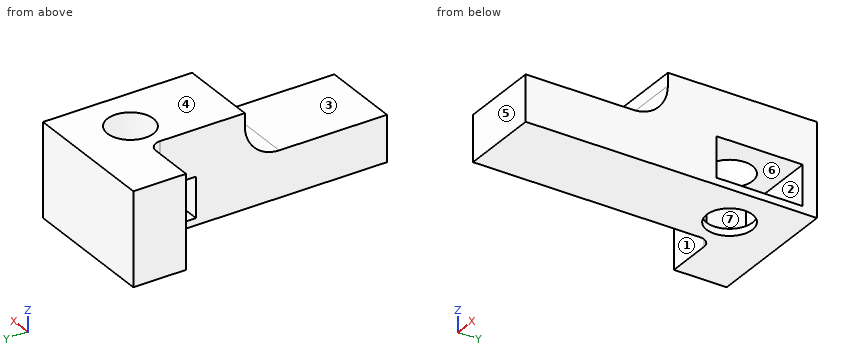
Autodesk Inventor part; units mm, degrees
ref_plane "Work Plane1" through (-21.8189, 29, 8.1) normal (0, 1, 0) x (0, 0, 1)
ref_plane "Work Plane2" through (-21.8189, 19, 8.1) normal (0, 0, -1) x (0, 1, 0)
ref_plane "YZ Plane" through (0, 0, 0) normal (1, 0, 0) x (0, 1, 0)
sketch "Sketch1" plane through (0, 0, 0) normal (0, 0, 1) x (1, 0, 0)
  line L0 (5.8439, -14.5) -> (6.8, -14.5)
  line L1 (6.8, -5.5) -> (6.8, -14.5)
  line L2 (6.8, -5.5) -> (5.8439, -5.5)
  arc A0 (5.8439, -3.1) -> (5.8439, -5.5) centre (4, -4.3) ccw
  line L3 (5.8439, -3.1) -> (6.8, -3.1)
  line L4 (6.8, 0) -> (6.8, -3.1)
  line L5 (0, 0) -> (6.8, 0)
  line L6 (0, -20) -> (0, 0)
  line L7 (0, -20) -> (6.8, -20)
  line L8 (6.8, -16.9) -> (6.8, -20)
  line L9 (6.8, -16.9) -> (5.8439, -16.9)
  arc A1 (5.8439, -14.5) -> (5.8439, -16.9) centre (4, -15.7) ccw
  line L10 (-47.1, -14.5) -> (-46.1439, -14.5)
  arc A2 (-46.1439, -16.9) -> (-46.1439, -14.5) centre (-44.3, -15.7) ccw
  line L11 (-46.1439, -16.9) -> (-47.1, -16.9)
  line L12 (-47.1, -16.9) -> (-47.1, -20)
  line L13 (-40.3, -20) -> (-47.1, -20)
  line L14 (-40.3, 0) -> (-40.3, -20)
  line L15 (-40.3, 0) -> (-47.1, 0)
  line L16 (-47.1, 0) -> (-47.1, -3.1)
  line L17 (-47.1, -3.1) -> (-46.1439, -3.1)
  arc A3 (-46.1439, -5.5) -> (-46.1439, -3.1) centre (-44.3, -4.3) ccw
  line L18 (-46.1439, -5.5) -> (-47.1, -5.5)
  line L19 (-47.1, -5.5) -> (-47.1, -14.5)
extrude "Extrusion1" add sketch "Sketch1" along normal blind 4
sketch "Sketch2" plane through (0, 0, 0) normal (0, 1, 0) x (1, 0, 0)
  line L0 (0, 0) -> (6.8, 0)
  line L1 (0, 0) -> (0, -4)
  line L2 (6.8, -4) -> (0, -4)
  line L3 (6.8, 0) -> (6.8, -4)
  line L4 (-47.1, 0) -> (-47.1, -4)
  line L5 (-40.3, -4) -> (-47.1, -4)
  line L6 (6.8, 0) -> (-47.1, 0)
  line L7 (-47.1, 0) -> (-47.1, -4)
  line L8 (-47.1, -4) -> (6.8, -4)
  line L9 (6.8, -4) -> (6.8, 0)
extrude "Extrusion2" add sketch "Sketch2" along normal blind 4 contours L1 L8 L5 L4 L6
sketch "Sketch3" plane through (0, 0, 4) normal (1, 0, 0) x (0, 0, -1)
  line L0 (4, 0) -> (0, 0)
  line L1 (4, 4) -> (4, 0)
  line L2 (0, 4) -> (4, 4)
  line L3 (0, 0) -> (0, 4)
extrude "Extrusion3" add sketch "Sketch3" along normal up to surface (6.8 mm away)
sketch "Sketch4" plane through (0, 4, 0) normal (0, 1, 0) x (1, 0, 0)
  line L0 (6.8, 0) -> (-47.1, 0)
  line L1 (-47.1, -4) -> (6.8, -4)
  line L2 (-9.3767, -8.1) -> (-9.3767, -13.1) construction
  line L3 (-21.8189, -8.1) -> (-9.3767, -8.1) construction
  arc A0 (-17.3767, -8.1) -> (-40.8, 16.4941) centre (-48.3, -14.1) ccw construction
  line L4 (-9.3767, -4) -> (-16.3767, -4) construction
  line L5 (-16.3767, -4) -> (-16.3767, -8.1) construction
  line L6 (-16.3767, -8.1) -> (-9.3767, -8.1) construction
  line L7 (-9.3767, -8.1) -> (-9.3767, -4) construction
  line L8 (-9.3767, -4) -> (-16.3767, -4)
  line L9 (-16.3767, -4) -> (-16.3767, 0)
  line L10 (-16.3767, 0) -> (-9.3767, 0)
  line L11 (-9.3767, 0) -> (-9.3767, -4)
  point P0 (0, 0)
  dimension "d6" = 7
ref_plane "Work Plane1" through (-21.8189, 29, 8.1) normal (0, 1, 0) x (0, 0, 1)
extrude "Extrusion4" add sketch "Sketch4" along normal up to surface (25 mm away)
sketch "Sketch5" plane through (0, 0, 4) normal (0, 0, 1) x (1, 0, 0)
  circle A0 centre (-13.3767, 24) radius 2 construction
  line L0 (-21.8189, 24) -> (-17.3767, 24) construction
  line L1 (-21.8189, 24) -> (-21.8189, 29) construction
  line L2 (-21.8189, 29) -> (-9.3767, 29) construction
  line L3 (-9.3767, 19) -> (-9.3767, 29) construction
  line L4 (-17.3767, 19) -> (-9.3767, 19) construction
  line L5 (-17.3767, 24) -> (-17.3767, 19) construction
  line L6 (-9.3767, 19) -> (-16.3767, 19) construction
  line L7 (-16.3767, 19) -> (-16.3767, 29) construction
  line L8 (-16.3767, 29) -> (-9.3767, 29) construction
  line L9 (-9.3767, 29) -> (-9.3767, 19) construction
  line L10 (-9.3767, 19) -> (-16.3767, 19)
  line L11 (-16.3767, 19) -> (-16.3767, 29)
  line L12 (-16.3767, 29) -> (-9.3767, 29)
  line L13 (-9.3767, 29) -> (-9.3767, 19)
  circle A1 centre (-13.3767, 24) radius 2
ref_plane "Work Plane2" through (-21.8189, 19, 8.1) normal (0, 0, -1) x (0, 1, 0)
extrude "Extrusion5" add sketch "Sketch5" along normal up to surface (4.1 mm away)
fillet "Fillet2" radius 2 2 edges at (-9.3767, 4, 2) (-16.3767, 4, 2)
sketch "Sketch6" plane through (-16.3767, 19, 8.1) normal (-1, 0, 0) x (0, 0, 1)
  line L0 (0, 5) -> (-24.5941, 5) construction
  line L1 (0, 0) -> (-24.5941, 0) construction
  line L2 (-8.1, 10) -> (0.5132, 10) construction
  line L3 (0.5132, 10) -> (0.5132, 5) construction
  line L4 (0.5132, 5) -> (-8.1, 5) construction
  line L5 (-8.1, 5) -> (-8.1, 10) construction
  line L6 (-8.1, 10) -> (0, 10)
  line L7 (0, 10) -> (0, 5)
  line L8 (0, 5) -> (-8.1, 5)
  line L9 (-8.1, 5) -> (-8.1, 10)
  point P0 (-8.1, -19)
extrude "Extrusion6" add sketch "Sketch6" along normal blind 5
sketch "Sketch7" plane through (-16.3767, 24, 0) normal (0, -1, 0) x (1, 0, 0)
  line L0 (0, 8.1) -> (0, 0)
  line L1 (0, 8.1) -> (-5, 8.1)
  line L2 (-5, 0) -> (-5, 8.1)
  line L3 (0, 0) -> (-5, 0)
  point P0 (16.3767, 0)
extrude "Extrusion7" cut sketch "Sketch7" against normal blind 0.4
sketch "Sketch8" plane through (0, 0, 0) normal (0, 0, -1) x (-1, 0, 0)
  circle A0 centre (13.3767, 24) radius 2 construction
  circle A1 centre (13.3767, 24) radius 2
extrude "Extrusion8" cut sketch "Sketch8" against normal blind 4
fillet "Fillet3" radius 1 1 edges at (-16.3767, 24.4, 4.05)
sketch "Sketch9" plane through (-9.3767, 19, 8.1) normal (1, 0, 0) x (0, 0, -1)
  line L0 (0, 0) -> (0, 10)
  line L1 (8.1, 7) -> (0, 7) construction
  line L2 (8.1, 3) -> (0, 3) construction
  line L3 (24.5941, 5) -> (0, 5) construction
  line L4 (-5, 5) -> (0, 5) construction
  line L5 (4, 8.75) -> (7.5, 8.75)
  line L6 (7.5, 8.75) -> (7.5, 1.25)
  line L7 (7.5, 1.25) -> (4, 1.25)
  line L8 (4, 1.25) -> (4, 8.75)
  point P0 (8.1, -19)
  point P1 (4, 5)
  dimension "d20" = 3.5
  dimension "d21" = 7.5
  dimension "d22" = 4
extrude "Extrusion9" cut sketch "Sketch9" against normal blind 7.5
sketch "Sketch10" plane through (-16.3767, 19, 4) normal (0, -1, 0) x (1, 0, 0)
  line L0 (0, 4.1) -> (7, 4.1)
  line L1 (0, 0) -> (0, 4.1)
  line L2 (7, 0) -> (0, 0)
  line L3 (7, 0) -> (7, 4.1)
  point P0 (16.3767, -4)
extrude "Extrusion10" add sketch "Sketch10" along normal blind 3
fillet "Fillet4" radius 3 1 edges at (-12.8767, 16, 4)
sketch "Sketch11" plane through (0, 0, 0) normal (0, -1, 0) x (1, 0, 0)
  line L0 (-40.3, 0) -> (-40.3, 4)
  line L1 (0, 0) -> (-40.3, 0)
  line L2 (0, 0) -> (0, 4)
  line L3 (-40.3, 4) -> (0, 4)
extrude "Extrusion11" cut sketch "Sketch11" against normal blind 0.3
sketch "Sketch12" plane through (0, -20, 0) normal (-1, 0, 0) x (0, 0, 1)
  line L0 (0, 0) -> (0, 20.3)
  line L1 (0, 0) -> (4, 0)
  line L2 (4, 20.3) -> (4, 0)
  line L3 (4, 20.3) -> (0, 20.3)
  point P0 (0, 20)
extrude "Extrusion12" cut sketch "Sketch12" against normal blind 0.3
sketch "Sketch13" plane through (-40.3, -20, 4) normal (1, 0, 0) x (0, 0, -1)
  line L0 (4, 0) -> (4, 20.3)
  line L1 (4, 20.3) -> (0, 20.3)
  line L2 (0, 0) -> (0, 20.3)
  line L3 (4, 0) -> (0, 0)
  point P0 (4, 20)
extrude "Extrusion13" cut sketch "Sketch13" against normal blind 0.3
fillet "Fillet5" radius 1 2 edges at (6.8, 4, 2) (-47.1, 4, 2)
sketch "Sketch15" plane through (0, 0, 4) normal (0, 0, 1) x (1, 0, 0)
  line L0 (-46.1, 4) -> (-18.3767, 4)
  line L1 (13.0867, -24.6558) -> (-51.2218, -24.6558)
  line L2 (-51.2218, -24.6558) -> (-51.2218, 7)
  line L3 (-51.2218, 7) -> (13.0867, 7)
  line L4 (13.0867, 7) -> (13.0867, -24.6558)
  point P0 (0, 0)
  dimension "d35" = 3
extrude "Extrusion14" cut sketch "Sketch15" against normal through all
sketch "Sketch16" plane through (-16.3767, 7, 4) normal (0, -1, 0) x (1, 0, 0)
  line L0 (7, 0) -> (7, -4)
  line L1 (0, 0) -> (7, 0)
  line L2 (0, -4) -> (0, 0)
  line L3 (7, -4) -> (0, -4)
  point P0 (16.3767, -4)
extrude "Extrusion15" add sketch "Sketch16" along normal blind 3.4
properties part number "MG996RBracketBottom"
Check sheet for the modelled part. Datum: model origin and axes. Units: mm. Face numbers are marked on the shaded views. A direction names the side the tool comes from. Give positions to 0.01 mm unless a question says otherwise; leave off trailing zeros. Order: outer loops, then holes, each group sorted by start corner. A loop starts at its lowest first (then second) coordinate and runs counter-clockwise, first axis right, second up. Notation, with made-up numbers: M -21.75,65.5 L 18.25,65.5 A20 ccw 18.25,100.5 Z; hole C 12.5,88.25 d6. An arc over 180 degrees is marked long. Answer in a Markdown table with one row per item. Add a question column.
Q1. Gauge pin test, flat ends, axial feed: pin 1 Ø1 at (y, z) = (10.5, 3) entering from -X; pin 2 Ø2 at (x, y) = (-14.5, 7) entering from +Z; pin 3 Ø1.5 at (x, z) = (-11, 6.5) entering from -Y; pin 4 Ø3 at (x, y) = (-18, 12.5) entering from -Z. Record the tip position at first contact, or that the pin passes through.
Q2. Sectioned sample at C-C, the plane y = 27.25. Record the boundary of the cut face in (x, z), and give its area (4 significant figures).
Q3. Release check for a two-part mould opening along Z. For the marked faces 4, 5, 6 and 7 record: released by +Z, released by -Z, zero draft, split by the parting line, or undercut.
Q4. Sectioned sample at A-A, the plane z = 3. Record the boundary of the cut face in (x, y).
Q5. Access from +Z, -Z, +X, -X, +Y, -Y to the whole of each face (thin tool, end or side, straight path). Record for the marked faces 1, 2 and 3.
Q6. Thickness scan on L1, parallel to Y at x = -9.75, z = 3.5; L2, parallel to Y at x = -13.25, z = 7.25; L3, parallel to Z at x = -16, y = 21.5. Record the ranges inside material, lowest first.
Q7. Sectioned sample at B-B, the plane z = 7.25. Record the boundary of the cut face in (x, y), and give its area (3 significant figures).
Q8. Sectioned sample at D-D, the plane y = 22.75. Record the boundary of the cut face in (x, z), and give its area (3 significant figures).
Verdict:
| question | item | result |
|---|---|---|
| 1 | pin 1 | x = -16.38 |
| 1 | pin 2 | z = 4 |
| 1 | pin 3 | y = 15.73 |
| 1 | pin 4 | through |
| 2 | outline | M -21.38,0 L -9.38,0 L -9.38,0.6 L -16.88,0.6 L -16.88,4.1 L -9.38,4.1 L -9.38,8.1 L -21.38,8.1 Z |
| 2 | area | 70.95 mm² |
| 3 | face 4 | released by +Z |
| 3 | face 5 | zero draft |
| 3 | face 6 | undercut |
| 3 | face 7 | undercut |
| 4 | outline | M -21.38,24.4 L -17.38,24.4 A1 cw -16.88,24.27 L -16.88,27.75 L -9.38,27.75 L -9.38,29 L -21.38,29 Z; M -16.38,3.6 L -9.38,3.6 L -9.38,20.25 L -16.38,20.25 Z |
| 5 | face 1 | +Z, -Z, -X, -Y |
| 5 | face 2 | +X |
| 5 | face 3 | +Z, +X, -X, -Y |
| 6 | L1 | 3.6 to 20.25, 27.75 to 29 |
| 6 | L2 | 16 to 22, 26 to 29 |
| 6 | L3 | 0 to 0.6, 4.1 to 8.1 |
| 7 | outline | M -21.38,24.4 L -17.38,24.4 A1 cw -16.38,23.4 L -16.38,16 L -9.38,16 L -9.38,29 L -21.38,29 Z; hole C -13.38,24 d4 |
| 7 | area | 102 mm² |
| 8 | outline | M -16.38,0 L -14.94,0 L -14.94,0.6 L -16.38,0.6 Z; M -16.38,4.1 L -14.94,4.1 L -14.94,8.1 L -16.38,8.1 Z; M -11.82,0 L -9.38,0 L -9.38,0.6 L -11.82,0.6 Z; M -11.82,4.1 L -9.38,4.1 L -9.38,8.1 L -11.82,8.1 Z |
| 8 | area | 17.8 mm² |
